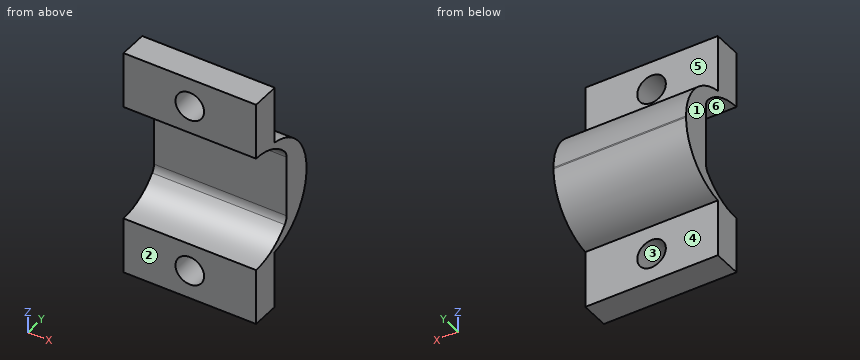
```python
from build123d import *

# Parameters (mm, degrees)
RESSALTO_EXTRUS_O1_DEPTH   = 15.9
FILETE1_R                  = 6
FILETE2_R                  = 1.2
CORTE_EXTRUS_O2_DEPTH      = 20.463298795
CORTE_EXTRUS_O2_DEPTH_BACK = 20.463298795
ESBO_O3_W                  = 2
ESBO_O3_H                  = 20.053518914
ESBO_O4_W                  = 13.9
ESBO_O4_H                  = 3
RESSALTO_EXTRUS_O2_DEPTH   = 2
ESBO_O5_W                  = 13.9
ESBO_O5_H                  = 3
RESSALTO_EXTRUS_O3_DEPTH   = 2
CORTE_EXTRUS_O3_DEPTH      = 10


with BuildPart() as part:
    # Esboço1 → Ressalto-extrusão1 (new body)
    with BuildSketch(Plane(origin=(0, 0, 0), x_dir=(0, 0, -1), z_dir=(1, 0, 0))):
        with BuildLine():
            ThreePointArc((-3.633180425, 4.9), (-1.913112647, 5.792236183), (0, 6.1))
            ThreePointArc((0, 6.1), (1.913112647, 5.792236183), (3.633180425, 4.9))
            ThreePointArc((3.633180425, 4.9), (5.448504409, 2.742954557), (6.1, 0))
            Line((6.1, 0), (10, 0))
            Line((10, 0), (10, 3))
            Line((10, 3), (6, 3))
            Line((6, 3), (6, 8.1))
            Line((6, 8.1), (-6, 8.1))
            Line((-6, 8.1), (-6, 3))
            Line((-6, 3), (-10, 3))
            Line((-10, 3), (-10, 0))
            Line((-10, 0), (-6.1, 0))
            ThreePointArc((-6.1, 0), (-5.448504409, 2.742954557), (-3.633180425, 4.9))
        make_face()
        with BuildLine():
            ThreePointArc((3.633180425, 4.9), (1.913112647, 5.792236183), (0, 6.1))
            Line((0, 6.1), (0, 4.9))
            Line((0, 4.9), (3.633180425, 4.9))
        make_face()
        with BuildLine():
            Line((0, 4.9), (0, 6.1))
            ThreePointArc((0, 6.1), (-1.913112647, 5.792236183), (-3.633180425, 4.9))
            Line((-3.633180425, 4.9), (0, 4.9))
        make_face()
    extrude(amount=RESSALTO_EXTRUS_O1_DEPTH)

    # Filete1
    # the kernel refuses this fillet: 6 mm, written as the material it takes off along each edge
    with BuildSketch(Plane(origin=(-14.83028995, 8.1, 6), x_dir=(0, -1, 0), z_dir=(1, 0, 0))) as filete1_piece_1:
        with BuildLine():
            CenterArc((6, 5.93211598), FILETE1_R, 180, 81.373073441)
            Line((0, 5.93211598), (-0.12, 5.93211598))
            Line((-0.12, 5.93211598), (-0.12, 0))
            Line((-0.12, 0), (0, -0.12))
            ThreePointArc((0, -0.12), (2.55, -0.12), (5.082, -0.11864232))
            Line((5.082, -0.11864232), (5.1, 0))
        make_face()
    extrude(amount=45.5605799, mode=Mode.SUBTRACT)
    with BuildSketch(Plane(origin=(-14.83028995, 8.1, -6), x_dir=(0, -1, 0), z_dir=(1, 0, 0))) as filete1_piece_2:
        with BuildLine():
            CenterArc((6, -5.93211598), FILETE1_R, 98.626926559, 81.373073441)
            Line((0, -5.93211598), (-0.12, -5.93211598))
            Line((-0.12, -5.93211598), (-0.12, 0))
            Line((-0.12, 0), (0, 0.12))
            ThreePointArc((0, 0.12), (2.55, 0.12), (5.082, 0.11864232))
            Line((5.082, 0.11864232), (5.1, 0))
        make_face()
    extrude(amount=45.5605799, mode=Mode.SUBTRACT)

    # Filete2
    filete2_edges = [part.edges().sort_by_distance(p)[0] for p in [
        (7.95, 4.9, -3.633180425),
        (7.95, 4.9, 3.633180425),
    ]]
    fillet(filete2_edges, radius=FILETE2_R)

    # Esboço3 → Corte-extrusão2 (cut, two sides: drawn at the far end of the back side and taken through both)
    with BuildSketch(Plane(origin=(0, 3, 0), x_dir=(1, 0, 0), z_dir=(0, 1, 0)).offset(-CORTE_EXTRUS_O2_DEPTH_BACK)):
        with Locations((1, -0.026759457)):
            Rectangle(ESBO_O3_W, ESBO_O3_H)
    extrude(amount=CORTE_EXTRUS_O2_DEPTH + CORTE_EXTRUS_O2_DEPTH_BACK, mode=Mode.SUBTRACT)

    # Esboço4 → Ressalto-extrusão2 (add)
    with BuildSketch(Plane.XY.offset(10)):
        with Locations((8.95, 1.5)):
            Rectangle(ESBO_O4_W, ESBO_O4_H)
    extrude(amount=RESSALTO_EXTRUS_O2_DEPTH)

    # Esboço5 → Ressalto-extrusão3 (add)
    with BuildSketch(Plane(origin=(0, 0, -10), x_dir=(-1, 0, 0), z_dir=(0, 0, -1))):
        with Locations((-8.95, 1.5)):
            Rectangle(ESBO_O5_W, ESBO_O5_H)
    extrude(amount=RESSALTO_EXTRUS_O3_DEPTH)

    # Esboço8 → Corte-extrusão3 (cut)
    with BuildSketch(Plane(origin=(0, 3, 0), x_dir=(1, 0, 0), z_dir=(0, 1, 0))):
        with BuildLine():
            ThreePointArc((10.45, 9), (8.95, 10.5), (7.45, 9))
            Line((7.45, 9), (10.45, 9))
        make_face()
        with BuildLine():
            Line((10.45, 9), (7.45, 9))
            ThreePointArc((7.45, 9), (8.95, 7.5), (10.45, 9))
        make_face()
        with BuildLine():
            ThreePointArc((10.45, -9), (8.95, -7.5), (7.45, -9))
            Line((7.45, -9), (10.45, -9))
        make_face()
        with BuildLine():
            Line((10.45, -9), (7.45, -9))
            ThreePointArc((7.45, -9), (8.95, -10.5), (10.45, -9))
        make_face()
    extrude(amount=-CORTE_EXTRUS_O3_DEPTH, mode=Mode.SUBTRACT)


solid = part.part
```
The listing builds one solid part. Answer for the finished solid, in the listing's coordinates (mm). Face numbers are marked on the shaded views. A direction names the side the tool comes from. Coordinates: 2 decimals unless noted, no trailing zeros. Write each loop counter-clockwise with the first axis right and the second up, starting at its lowest first coordinate (ties: lowest second). Pieces come first, ordered by that corner, then holes.
Q1. Find the intervals of material crossed by line 1 along Z through (x, y) = (8.95, 2.3); line 2 along Y through (x, z) = (11.75, 9.75); line 3 along Z through (x, y) = (8.95, 2.1), in increasing order.
Returned:
line 1: z = -12 to -10.5, -7.5 to -5.65, 5.65 to 7.5, 10.5 to 12
line 2: y = 0 to 3
line 3: z = -12 to -10.5, -7.5 to -5.73, 5.73 to 7.5, 10.5 to 12
Q2. Section A-A, the plane z = -9 is taken. Write down the section's boundary in (x, y).
Returned:
outline: (2, 0) - (7.45, 0) - (7.45, 3) - (2, 3) - close; (10.45, 0) - (15.9, 0) - (15.9, 3) - (10.45, 3) - close
Q3. Section D-D, the plane y = 4.25 is taken. Write down the section's boundary in (x, z), then the cut area to 3 significant figures.
Returned:
outline: (2, -5.67) - (15.9, -5.67) - (15.9, -4.38) - (2, -4.38) - close; (2, 4.38) - (15.9, 4.38) - (15.9, 5.67) - (2, 5.67) - close
area: 36.0 mm2
Q4. Which of the six approach directions +Z, -Z, +X, -X, +Y, -Y give full straight-line access (tool end or side, diameter ignored) to the marked faces 4, 5 and 6?
Returned:
face 4: -Z, +X, -X, +Y
face 5: +Z, +X, -X, +Y
face 6: +X, -X, -Y
Q5. Given P1, Ø5, axis at x = 6.5, z = 1, coming from the -Y side; P2, Ø3, axis at x = 8.5, z = 8, coming from the +Y side; P3, Ø1, axis at x = 12.5, z = -3, coming from the +Y side, each flat-ended and moving along its own axis, determine where each tip first touches the part or whether it passes through.
Returned:
P1: stops at y = 4.87
P2: stops at y = 3
P3: stops at y = 7.58
Q6. Section C-C, the plane x = 8.95 is taken. Write down the section's boundary in (y, z).
Returned:
outline: (0, -12) - (3, -12) - (3, -10.5) - (0, -10.5) - close; (0, -7.5) - (3, -7.5) - (3, -6) arc R6 ccw to (8.1, -0.07) - (8.1, 0.07) arc R6 ccw to (3, 6) - (3, 7.5) - (0, 7.5) - (0, 6.1) arc R6.1 cw to (4.61, 4) arc R1.2 cw to (4.9, 3.21) - (4.9, -3.21) arc R1.2 cw to (4.61, -4) arc R6.1 cw to (0, -6.1) - close; (0, 10.5) - (3, 10.5) - (3, 12) - (0, 12) - close
Q7. Section B-B, the plane y = 1 is taken. Write down the section's boundary in (x, z), then the cut area to 3 significant figures.
Returned:
outline: (2, -12) - (15.9, -12) - (15.9, -6.02) - (2, -6.02) - close; (2, 6.02) - (15.9, 6.02) - (15.9, 12) - (2, 12) - close; hole circle Ø3 at (8.95, -9); hole circle Ø3 at (8.95, 9)
area: 152 mm2
Q8. The mould has two halves that part along X. Classify the marked faces 1, 2 and 3: released by +X, released by -X, zero draft, split by the parting line, or undercut.
Returned:
face 1: released by -X
face 2: zero draft
face 3: undercut
